Build history of the part. All positions in model axes, mm. Round coordinates to 2 decimals unless told otherwise and drop trailing zeros. Write each loop counter-clockwise with the first axis right and the second up, starting at its lowest first coordinate (ties: lowest second). Pieces come first, ordered by that corner, then holes.
1) Saw through at C-C (x = 35). Write the cut outline in (y, z), plus the area to 3 significant figures.
2) Wall check: probe 1 along Y at (x, z) = (-50, 1.85); probe 2 along Y at (x, z) = (35, 0.45); probe 3 along Y at (x, z) = (0, 1.65). Give the ranges that are in metal, low to high.
3) Saw through at B-B (z = 1.9). State how many separate pieces and enclosed holes the cut face has, plus the area to 3 significant figures.
4) Saw through at D-D (y = -6.5). Write the cut outline in (x, z).
5) Saw through at A-A (x = 0). Write the cut outline in (y, z).
6) Pull direction X, two halves, no side cores. Call faces 1 (the conical face through (-34.179, 3.892, 0.984)), 2 (the cylindrical face through (-35.78, -8.98, 0.42)), 3 (the cylindrical face through (-59.4, 19.43, 1.52)), 4 (the flat face through (60, 0, 1)): +X half, -X half, draft (parallel to the pull), parting line (faces both ways), or undercut.
7) Flat gauge pin, fed straight in: pin 1 (5 mm diameter, centred on x = 50, y = -11, fed in from -Z). Where does the tip first touch, or does it go through?
Autodesk Fusion 360 part; units mm, degrees
sketch "Boceto1" plane through (0, 0, 0) normal (0, 0, 1) x (1, 0, 0)
  line L0 (60, -20) -> (-60, -20)
  line L1 (-60, -20) -> (-60, 20)
  line L2 (-60, 20) -> (60, 20)
  line L3 (60, 20) -> (60, -20)
  line L4 (60, -20) -> (-60, 20) construction
  line L5 (-60, -20) -> (60, 20) construction
  circle A0 centre (0, 0) radius 9.5
  circle A1 centre (-50, 11) radius 3
  circle A2 centre (50, 11) radius 3
  circle A3 centre (-50, -11) radius 3
  circle A4 centre (50, -11) radius 3
  dimension "d1" = 120
  dimension "d2" = 40
  dimension "d3" = 19
  dimension "d4" = 6
  dimension "d5" = 10
  dimension "d6" = 11
  dimension "d9" = 100
  dimension "d10" = -22
extrude "Extruir1" add sketch "Boceto1" along normal blind 3
sketch "Boceto2" plane through (0, 0, 3) normal (0, 0, 1) x (-1, 0, 0)
  circle A0 centre (0, 0) radius 9.5
  circle A1 centre (-50, -11) radius 3
  circle A2 centre (-50, 11) radius 3
  circle A3 centre (50, -11) radius 3
  circle A4 centre (50, 11) radius 3
  line L0 (-60, -20) -> (60, -20)
  line L1 (60, -20) -> (60, 20)
  line L2 (60, 20) -> (-60, 20)
  line L3 (-60, 20) -> (-60, -20)
  line L4 (35, -6.5) -> (-35, -6.5) construction
  line L5 (-35, -6.5) -> (-35, 6.5) construction
  line L6 (-35, 6.5) -> (35, 6.5) construction
  line L7 (35, 6.5) -> (35, -6.5) construction
  line L8 (35, -6.5) -> (-35, 6.5) construction
  line L9 (-35, -6.5) -> (35, 6.5) construction
  point P0 (35, -6.5)
  point P1 (35, 6.5)
  point P2 (-35, 6.5)
  point P3 (-35, -6.5)
  dimension "d18" = 13
  dimension "d19" = 25
hole "Agujero2" at (35, 6.5, 3) at (-35, 6.5, 3) at (-35, -6.5, 3) at (35, -6.5, 3) direction (0, 0, -1) diameter 5.2 depth 15 tip angle 180 countersink diameter 9.5 countersink angle 90
fillet "Empalme1" radius 2 4 edges at (-60, -20, 1.5) (-60, 20, 1.5) (60, -20, 1.5) (60, 20, 1.5)
Evaluation:
1. outline: (-20, 0) - (-9.1, 0) - (-9.1, 0.85) - (-11.25, 3) - (-20, 3) - close; (-3.9, 0) - (3.9, 0) - (3.9, 0.85) - (1.75, 3) - (-1.75, 3) - (-3.9, 0.85) - close; (9.1, 0) - (20, 0) - (20, 3) - (11.25, 3) - (9.1, 0.85) - close
1. area: 79.6 mm2
2. probe 1: y = -20 to -14, -8 to 8, 14 to 20
2. probe 2: y = -20 to -9.1, -3.9 to 3.9, 9.1 to 20
2. probe 3: y = -20 to -9.5, 9.5 to 20
3. separate pieces: 1
3. enclosed holes: 9
3. area: 4,230 mm2
4. outline: (-60, 0) - (-37.6, 0) - (-37.6, 0.85) - (-39.75, 3) - (-60, 3) - close; (-32.4, 0) - (-6.93, 0) - (-6.93, 3) - (-30.25, 3) - (-32.4, 0.85) - close; (6.93, 0) - (32.4, 0) - (32.4, 0.85) - (30.25, 3) - (6.93, 3) - close; (37.6, 0) - (60, 0) - (60, 3) - (39.75, 3) - (37.6, 0.85) - close
5. outline: (-20, 0) - (-9.5, 0) - (-9.5, 3) - (-20, 3) - close; (9.5, 0) - (20, 0) - (20, 3) - (9.5, 3) - close
6. face 1: undercut
6. face 2: undercut
6. face 3: -X half
6. face 4: +X half
7. pin 1: passes through
